Autodesk Inventor part; units mm, degrees
ref_plane "YZ Plane" through (0, 0, 0) normal (1, 0, 0) x (0, 1, 0)
ref_plane "XZ Plane" through (0, 0, 0) normal (0, 1, 0) x (-1, 0, 0)
ref_plane "XY Plane" through (0, 0, 0) normal (0, 0, 1) x (1, 0, 0)
sketch "Sketch1" plane through (0, 0, 0) normal (0, 1, 0) x (-1, 0, 0)
  line L0 (10, 0) -> (80, 0)
  line L1 (90, -32.6619) -> (90, -167.3381)
  line L2 (67, -200) -> (23, -200)
  line L3 (0, -167.3381) -> (0, -85)
  line L4 (22, -27) -> (68, -27) construction
  line L5 (68, -27) -> (68, -173) construction
  line L6 (68, -173) -> (22, -173) construction
  circle A0 centre (68, -27) radius 1.5
  circle A1 centre (68, -173) radius 1.5
  circle A2 centre (22, -173) radius 1.5
  circle A3 centre (22, -27) radius 1.5
  line L7 (30, -70) -> (60, -70)
  line L8 (70, -80) -> (70, -120)
  line L9 (60, -130) -> (30, -130)
  line L10 (20, -120) -> (20, -80)
  arc A4 (70, -80) -> (60, -70) centre (60, -80) ccw
  arc A5 (60, -130) -> (70, -120) centre (60, -120) ccw
  arc A6 (20, -120) -> (30, -130) centre (30, -120) ccw
  arc A7 (30, -70) -> (20, -80) centre (30, -80) ccw
  arc A8 (90, -10) -> (80, 0) centre (80, -10) ccw
  arc A9 (0, -190) -> (10, -200) centre (10, -190) ccw
  arc A10 (80, -200) -> (90, -190) centre (80, -190) ccw
  arc A11 (10, 0) -> (0, -10) centre (10, -10) ccw
  circle A12 centre (80, -10) radius 1.25
  circle A13 centre (80, -30) radius 1.25
  circle A14 centre (80, -50) radius 1.25
  circle A15 centre (80, -70) radius 1.25
  circle A16 centre (80, -90) radius 1.25
  circle A17 centre (80, -110) radius 1.25
  circle A18 centre (80, -130) radius 1.25
  circle A19 centre (80, -150) radius 1.25
  circle A20 centre (80, -170) radius 1.25
  circle A21 centre (80, -190) radius 1.25
  circle A22 centre (10, -10) radius 1.25
  circle A23 centre (10, -30) radius 1.25
  circle A24 centre (10, -50) radius 1.25
  circle A25 centre (10, -70) radius 1.25
  circle A26 centre (10, -90) radius 1.25
  circle A27 centre (10, -110) radius 1.25
  circle A28 centre (10, -130) radius 1.25
  circle A29 centre (10, -150) radius 1.25
  circle A30 centre (10, -170) radius 1.25
  circle A31 centre (10, -190) radius 1.25
  circle A32 centre (81, -111) radius 3.5
  circle A33 centre (81.25, -89) radius 3.5
  circle A34 centre (9, -111) radius 3.5
  circle A35 centre (9, -89) radius 3.5
  line L11 (85.145, -24.087) -> (64.0418, -11.4251)
  line L12 (12.8542, -19.2875) -> (25.9582, -11.4251)
  arc A36 (90, -32.6619) -> (85.145, -24.087) centre (80, -32.6619) ccw
  arc A37 (4.855, -24.087) -> (0, -32.6619) centre (10, -32.6619) ccw construction
  circle A38 centre (67.5, -65) radius 1.25
  circle A39 centre (22.5, -65) radius 1.25
  line L13 (-15, -70) -> (15, -70) construction
  circle A40 centre (67.5, -20) radius 1.25
  line L14 (30, -25) -> (60, -25) construction
  circle A41 centre (22.5, -20) radius 1.25
  line L15 (-15, -25) -> (15, -25) construction
  line L16 (58.8968, -10) -> (31.1032, -10)
  arc A42 (64.0418, -11.4251) -> (58.8968, -10) centre (58.8968, -20) ccw
  arc A43 (31.1032, -10) -> (25.9582, -11.4251) centre (31.1032, -20) ccw
  line L17 (90, -200) -> (72, -200) construction
  line L18 (72, -195) -> (72, -185)
  line L19 (77, -180) -> (85, -180)
  line L20 (90, -175) -> (90, -167.3381)
  line L21 (0, -200) -> (18, -200) construction
  line L22 (18, -195) -> (18, -185)
  line L23 (13, -180) -> (5, -180)
  line L24 (0, -175) -> (0, -167.3381)
  arc A44 (77, -180) -> (72, -185) centre (77, -185) ccw
  arc A45 (85, -180) -> (90, -175) centre (85, -175) ccw
  arc A46 (0, -175) -> (5, -180) centre (5, -175) ccw
  arc A47 (18, -185) -> (13, -180) centre (13, -185) ccw
  arc A48 (67, -200) -> (72, -195) centre (67, -195) ccw
  arc A49 (18, -195) -> (23, -200) centre (23, -195) ccw
  circle A50 centre (69.1385, -144.2) radius 1.25
  circle A51 centre (20.8615, -144.2) radius 1.25
  circle A52 centre (53.8985, -195) radius 1.25
  line L25 (10, -30) -> (-10, -30) construction
  line L26 (-10, -30) -> (-10, -50) construction
  circle A53 centre (-10, -50) radius 1.25
  circle A54 centre (-10, -30) radius 1.25
  line L27 (-10, -30) -> (-10, -20) construction
  line L28 (-10, -20) -> (10.2817, -20)
  line L29 (-10, -20) -> (-15, -20)
  line L30 (-20, -25) -> (-20, -75)
  line L31 (-15, -80) -> (-5, -80)
  arc A55 (0, -85) -> (-5, -80) centre (-5, -85) ccw
  arc A56 (10.2817, -20) -> (12.8542, -19.2875) centre (10.2817, -15) ccw
  arc A57 (-15, -20) -> (-20, -25) centre (-15, -25) ccw
  arc A58 (-20, -75) -> (-15, -80) centre (-15, -75) ccw
  circle A59 centre (-10, -70) radius 1.25
  line L32 (10, -70) -> (-10, -50) construction
  line L33 (-10, -50) -> (10, -30) construction
  circle A60 centre (0, -60) radius 7.5
  circle A61 centre (0, -40) radius 7.5
  line L34 (67.5, -65) -> (22.5, -20) construction
  circle A62 centre (45, -42.5) radius 15
  line L35 (69.1385, -144.2) -> (22, -173) construction
  circle A63 centre (45, -158.9478) radius 15
  point P0 (0, 0)
  point P1 (90, 0)
  point P2 (70, -130)
  point P3 (70, -70)
  point P4 (20, -130)
  point P5 (45, 0)
  point P6 (45, -200)
  point P7 (25, -70)
  point P8 (70, -25)
  point P9 (25, -25)
  point P10 (72, -180)
  point P11 (-20, -20)
  point P12 (-20, -80)
  dimension "d0" = 90
  dimension "d1" = 200
  dimension "d2" = 46
  dimension "d4" = 22
  dimension "d5" = 27
  dimension "d6" = 3
  dimension "d7" = 3
  dimension "d8" = 3
  dimension "d9" = 3
  dimension "d10" = 50
  dimension "d11" = 60
  dimension "d12" = 20
  dimension "d13" = 70
  dimension "d14" = 10
  dimension "d15" = 10
  dimension "d16" = 2.5
  dimension "d19" = 20
  dimension "d24" = 2.5
  dimension "d27" = 20
  dimension "d34" = 7
  dimension "d35" = 7
  dimension "d36" = 7
  dimension "d37" = 7
  dimension "d38" = 72
  dimension "d39" = 22
  dimension "d40" = 9
  dimension "d41" = 89
  dimension "d42" = 22
  dimension "d43" = 72
  dimension "d46" = 10
  dimension "d48" = 2.5
  dimension "d51" = 45
  dimension "d54" = 45
  dimension "d57" = 22.5
  dimension "d58" = 5
  dimension "d59" = 10
  dimension "d71" = 18
  dimension "d72" = 20
  dimension "d73" = 18
  dimension "d74" = 5
  dimension "d75" = 5
  dimension "d76" = 2.5
  dimension "d77" = 2.5
  dimension "d78" = 0
  dimension "d79" = 48.277
  dimension "d81" = 20.8615
  dimension "d82" = 2.5
  dimension "d83" = 15.24
  dimension "d84" = 50.8
  dimension "d85" = 5
  dimension "d86" = 20
  dimension "d87" = 20
  dimension "d88" = 2.5
  dimension "d89" = 2.5
  dimension "d90" = 10
  dimension "d91" = 10
  dimension "d92" = 60
  dimension "d93" = 5
  dimension "d94" = 2.5
  dimension "d95" = 15
  dimension "d97" = 30
  dimension "d98" = 30
extrude "Extrusion2" add sketch "Sketch1" along normal blind 3 contours L1 L20 A45 L19 A44 L18 A48 L2 A49 L22 A47 L23 A46 L24 L3 A55 L31 A58 L30 A57 L29 L28 A56 L12 A43 L16 A42 L11 A36
equation "\"d4\" = -0.5 * d2 + 0.5 * d0"
equation "\"d5\" = -0.5 * d3 + 0.5 * d1"
equation "\"d12\" = -0.5 * d10 + 0.5 * d0"
equation "\"d13\" = -0.5 * d11 + 0.5 * d1"
equation "\"d40\" = -0.5 * d38 + 0.5 * d0"
equation "\"d41\" = -0.5 * d39 + 0.5 * d1"
equation "\"d57\" = -0.5 * d51 + 0.5 * d0"
equation "\"d81\" = -0.5 * d79 + 0.5 * d0"
properties part number "ElectronicsBaseplateV01" material "Polycarbonate, Clear"
Geometry check sheet. Reference: the model listing, model coordinates, mm. A direction names the side the tool comes from. Give positions to 0.01 mm unless a question says otherwise; leave off trailing zeros. Write each loop counter-clockwise with the first axis right and the second up, starting at its lowest first coordinate (ties: lowest second). Pieces come first, ordered by that corner, then holes.
1) Release check for a two-part mould opening along Z. For faces 1 (the face through (0.976, 1.479, -67.436)), 2 (the face through (-75, 1, -18)), 3 (the face through (2, 1, -81)) record: released by +Z, released by -Z, zero draft, split by the parting line, or undercut.
Values follow:
face 1: undercut
face 2: released by +Z
face 3: released by -Z
2) Cross-section at D-D (x = -16). Record the boundary of the cut face in (y, z).
Values follow:
outline: (0, -181) - (3, -181) - (3, -17.4) - (0, -17.4) - close
3) Set-up check for faces 4 (the face through (-89, 1, -178)), 5 (the face through (-22.85, 1.48, -73.01)): record each of +Z, -Z, +X, -X, +Y, -Y from which the full face is reachable in a straight line by a thin tool's end or side.
Values follow:
face 4: -Z, -X, +Y, -Y
face 5: +Y, -Y
4) Go/stop test with flat-tipped pins: pin 1 Ø0.9 at (x, y) = (-81.5, 1.5) entering from -Z; pin 2 Ø1.5 at (x, z) = (-22.5, -20) entering from -Y; pin 3 Ø0.9 at (y, z) = (1, -149) entering from +X. Record where each tip stops, or that it passes through.
Values follow:
pin 1: stops at z = -180
pin 2: passes through
pin 3: stops at x = 0
5) Cross-section at C-C (z = -162.5). Record the boundary of the cut face in (x, y), plus the area to 3 significant figures.
Values follow:
outline: (-90, 0) - (-59.57, 0) - (-59.57, 3) - (-90, 3) - close; (-30.43, 0) - (0, 0) - (0, 3) - (-30.43, 3) - close
area: 183 mm2
6) Cross-section at A-A (z = -82). Record the boundary of the cut face in (x, y), plus the area to 3 significant figures.
Values follow:
outline: (-90, 0) - (-70, 0) - (-70, 3) - (-90, 3) - close; (-20, 0) - (1, 0) - (1, 3) - (-20, 3) - close
area: 123 mm2
7) Cross-section at B-B (x = -44). Record the boundary of the cut face in (y, z).
Values follow:
outline: (0, -200) - (3, -200) - (3, -173.91) - (0, -173.91) - close; (0, -143.98) - (3, -143.98) - (3, -130) - (0, -130) - close; (0, -70) - (3, -70) - (3, -57.47) - (0, -57.47) - close; (0, -27.53) - (3, -27.53) - (3, -10) - (0, -10) - close
8) Thickness scan on line 1 (Z direction, x = -2, y = 2.85); line 2 (X direction, y = 2.35, z = -105.5); line 3 (X direction, y = 2.4, z = -158.5). Record the ranges inside material, lowest first.
Values follow:
line 1: z = -179 to -67.23, -52.77 to -47.23, -32.77 to -20
line 2: x = -90 to -70, -20 to 0
line 3: x = -90 to -59.99, -30.01 to 0
